Read the model definition and answer for the solid it produces. Units are mm, in the model's axes. A direction names the side the tool comes from. Coordinates: 2 decimals unless noted, no trailing zeros. Loops run counter-clockwise (first coordinate to the right, second up) from the corner with the lowest first, then second, coordinate; pieces in that order, holes last.
Q1. Section C-C (z = 7.25) is taken. Give the vertices of the cut face in (x, y), then the cut area to 3 significant figures.
Q2. Which of the six approach directions +Z, -Z, +X, -X, +Y, -Y give full straight-line access (tool end or side, diameter ignored) to faces 1 (the face through (-17, 0.5, 6)), 2 (the face through (17, 0.5, -6)), 3 (the face through (-17, 0.5, -6)), 4 (the face through (17, 0.5, 6))?
Q3. Section B-B (x = 6.5) is taken. Give the vertices of the cut face in (y, z).
Q4. Straight lines are drawn through the part: line 1 (Y direction, x = -1, z = 2.25); line 2 (X direction, y = 1.6, z = 2.5); line 3 (X direction, y = 0.85, z = 6.25). For each, find the intervals that lie inside material, in ascending order.
Q5. Section D-D (z = -5.5) is taken. Give the vertices of the cut face in (x, y).
Q6. Flat-ended cylindrical pins translate along their axes: P1, Ø8, axis at x = -8.5, z = -5, coming from the +Y side; P2, Ø0.5, axis at x = 11.5, y = 1.5, coming from the +Z side. Find the tip coordinate at first contact, or state that the pin passes through.
Q7. Section A-A (y = 0.4) is taken. Give the vertices of the cut face in (x, z), then the cut area to 3 significant figures.
from build123d import *

# Parameters (mm, degrees)
ESTRUSIONE_ESTRUSIONE1_DEPTH = 1
SCHIZZO2_W                   = 7
SCHIZZO2_H                   = 9
ESTRUSIONE_ESTRUSIONE2_DEPTH = 1
RACCORDO2_R                  = 0.5
RACCORDO3_R                  = 0.25
SCHIZZO4_W                   = 1
SCHIZZO4_H                   = 8
ESTRUSIONE_ESTRUSIONE6_DEPTH = 0.2
ESTRUSIONE_ESTRUSIONE7_DEPTH = 8
SCHIZZO6_W                   = 1.5
SCHIZZO6_H                   = 0.5
SCHIZZO6_H_2                 = 0.25
TAGLIO_ESTRUSIONE1_DEPTH     = 1
RACCORDO6_R                  = 0.1
RACCORDO6_OF_SPECCHIA1_R     = 0.1


with BuildPart() as part:
    # Schizzo1 → Estrusione-Estrusione1 (new body)
    with BuildSketch(Plane(origin=(0, 0, 0), x_dir=(1, 0, 0), z_dir=(0, 1, 0))):
        Polygon((-16, -8), (-16, -6), (-18, -6), (-18, 6), (-16, 6), (-16, 8), (16, 8), (16, 6), (18, 6), (18, -6), (16, -6), (16, -8), align=None)
    extrude(amount=ESTRUSIONE_ESTRUSIONE1_DEPTH)

    # Schizzo2 → Estrusione-Estrusione2 (add)
    with BuildSketch(Plane(origin=(0, 1, 0), x_dir=(1, 0, 0), z_dir=(0, 1, 0))):
        with Locations((7, 0)):
            Rectangle(SCHIZZO2_W, SCHIZZO2_H)
    extrude(amount=ESTRUSIONE_ESTRUSIONE2_DEPTH)

    # Raccordo2
    raccordo2_edges = [part.edges().sort_by_distance(p)[0] for p in [
        (10.5, 1.5, 4.5),
        (10.5, 1.5, -4.5),
        (3.5, 1.5, -4.5),
        (3.5, 1.5, 4.5),
    ]]
    fillet(raccordo2_edges, radius=RACCORDO2_R)

    # Raccordo3
    raccordo3_edges = [part.edges().sort_by_distance(p)[0] for p in [
        (3.5, 2, 0),
        (7, 2, -4.5),
        (10.5, 2, 0),
        (7, 2, 4.5),
        (3.646446609, 2, 4.353553391),
        (10.353553391, 2, 4.353553391),
        (10.353553391, 2, -4.353553391),
        (3.646446609, 2, -4.353553391),
    ]]
    fillet(raccordo3_edges, radius=RACCORDO3_R)

    # Schizzo4 → Estrusione-Estrusione6 (add)
    with BuildSketch(Plane(origin=(0, 1, 0), x_dir=(1, 0, 0), z_dir=(0, 1, 0))):
        with Locations((2.5, 0)):
            Rectangle(SCHIZZO4_W, SCHIZZO4_H)
    estrusione_estrusione6 = extrude(amount=ESTRUSIONE_ESTRUSIONE6_DEPTH)

    # Schizzo5 → Estrusione-Estrusione7 (add)
    with BuildSketch(Plane.XY.offset(4)):
        Polygon((3, 1), (3, 1.2), (3.5, 1.488675135), (3.5, 1.288675135), align=None)
    estrusione_estrusione7 = extrude(amount=-ESTRUSIONE_ESTRUSIONE7_DEPTH)

    # Schizzo6 → Taglio-Estrusione1 (cut)
    with BuildSketch(Plane(origin=(0, 1, 0), x_dir=(1, 0, 0), z_dir=(0, 1, 0))):
        with Locations((2.75, -3)):
            Rectangle(SCHIZZO6_W, SCHIZZO6_H)
        with Locations((2.75, -2)):
            Rectangle(SCHIZZO6_W, SCHIZZO6_H)
        with Locations((2.75, -1)):
            Rectangle(SCHIZZO6_W, SCHIZZO6_H)
        with Locations((2.75, 0)):
            Rectangle(SCHIZZO6_W, SCHIZZO6_H)
        with Locations((2.75, 1)):
            Rectangle(SCHIZZO6_W, SCHIZZO6_H)
        with Locations((2.75, 2)):
            Rectangle(SCHIZZO6_W, SCHIZZO6_H)
        with Locations((2.75, 3)):
            Rectangle(SCHIZZO6_W, SCHIZZO6_H)
        with Locations((2.75, 3.875)):
            Rectangle(SCHIZZO6_W, SCHIZZO6_H_2)
        with Locations((2.75, -3.875)):
            Rectangle(SCHIZZO6_W, SCHIZZO6_H_2)
    taglio_estrusione1 = extrude(amount=TAGLIO_ESTRUSIONE1_DEPTH, mode=Mode.SUBTRACT)

    # Raccordo6
    raccordo6_edges = [part.edges().sort_by_distance(p)[0] for p in [
        (2, 1.1, 1.75),
        (2, 1.1, 2.25),
        (2, 1.1, 0.75),
        (2, 1.1, 1.25),
        (2, 1.1, -0.25),
        (2, 1.1, 0.25),
        (2, 1.1, -1.25),
        (2, 1.1, -0.75),
        (2, 1.1, 3.75),
        (2, 1.1, -3.75),
        (2, 1.1, -3.25),
        (2, 1.1, -2.75),
        (2, 1.1, -2.25),
        (2, 1.1, -1.75),
        (2, 1.1, 2.75),
        (2, 1.1, 3.25),
    ]]
    fillet(raccordo6_edges, radius=RACCORDO6_R)

    # Specchia1: Estrusione-Estrusione6, Estrusione-Estrusione7, Taglio-Estrusione1 across plane
    add(estrusione_estrusione6.mirror(Plane.ZY.offset(-7)))
    add(estrusione_estrusione7.mirror(Plane.ZY.offset(-7)))
    add(taglio_estrusione1.mirror(Plane.ZY.offset(-7)), mode=Mode.SUBTRACT)

    # Raccordo6 of Specchia1
    raccordo6_of_specchia1_edges = [part.edges().sort_by_distance(p)[0] for p in [
        (12, 1.1, 1.75),
        (12, 1.1, 2.25),
        (12, 1.1, 0.75),
        (12, 1.1, 1.25),
        (12, 1.1, -0.25),
        (12, 1.1, 0.25),
        (12, 1.1, -1.25),
        (12, 1.1, -0.75),
        (12, 1.1, 3.75),
        (12, 1.1, -3.75),
        (12, 1.1, -3.25),
        (12, 1.1, -2.75),
        (12, 1.1, -2.25),
        (12, 1.1, -1.75),
        (12, 1.1, 2.75),
        (12, 1.1, 3.25),
    ]]
    fillet(raccordo6_of_specchia1_edges, radius=RACCORDO6_OF_SPECCHIA1_R)


solid = part.part
Numbers:
1. outline: (-16, 0) - (16, 0) - (16, 1) - (-16, 1) - close
1. area: 32.0 mm2
2. face 1: +Z, -X, +Y, -Y
2. face 2: -Z, +X, +Y, -Y
2. face 3: -Z, -X, +Y, -Y
2. face 4: +Z, +X, +Y, -Y
3. outline: (0, -8) - (1, -8) - (1, -4.5) - (1.75, -4.5) arc R0.25 ccw to (2, -4.25) - (2, 4.25) arc R0.25 ccw to (1.75, 4.5) - (1, 4.5) - (1, 8) - (0, 8) - close
4. line 1: y = 0 to 1
4. line 2: x = 3.5 to 10.5
4. line 3: x = -16 to 16
5. outline: (-18, 0) - (18, 0) - (18, 1) - (-18, 1) - close
6. P1: stops at y = 1
6. P2: passes through
7. outline: (-18, -6) - (-16, -6) - (-16, -8) - (16, -8) - (16, -6) - (18, -6) - (18, 6) - (16, 6) - (16, 8) - (-16, 8) - (-16, 6) - (-18, 6) - close
7. area: 560 mm2
